The figure shows three views and two pictorial views of one solid part (mm, origin at its lowest corner). Answer the questions. A direction names the side the tool comes from. Give positions to 0.01 mm unless a question says otherwise; leave off trailing zeros. Write each loop counter-clockwise with the first axis right and the second up, starting at its lowest first coordinate (ties: lowest second). Pieces come first, ordered by that corner, then holes. Notation, with made-up numbers: (76, -16.5) -> (102, -16.5) arc R23 cw to (102, -0.5) -> close; hole circle Ø6 at (31, 26). An arc over 180 degrees is marked (long way). Answer as CSV lines item,"result". Start each with the question number.
1. The part is cut by section B-B, the plane x = 40. Determine the outline of the cut face in (y, z), and give its area (3 significant figures).
2. The part is cut by section A-A, the plane y = 40. Determine the outline of the cut face in (x, z).
3. The part is cut by section C-C, the plane z = 2. Determine the outline of the cut face in (x, y).
4. Given pin 1 (4 mm diameter, centred on x = 60.5, z = 7.5, fed in from +Y); pin 2 (8 mm diameter, centred on x = 49.5, y = 11, fed in from +Z); pin 3 (10 mm diameter, centred on x = 66, z = 3.5, fed in from -Y), each flat-ended and moving along its own axis, determine where each tip first touches the part or whether it passes through.
5. A tool of negligible diameter and unlimited length cuts with its end or side. For the marked faces 1 and 2, from which of +Z, -Z, +X, -X, +Y, -Y can it reach the whole face along a straight path? Write none if from no direction.
6. Find the intervals of material crossed by line 1 (Y direction, x = 40, z = 7.5); line 2 (Z direction, x = 40, y = 35); line 3 (Z direction, x = 74, y = 21), in increasing order.
7. The part is cut by section D-D, the plane x = 20. Determine the outline of the cut face in (y, z), and give its area (4 significant figures).
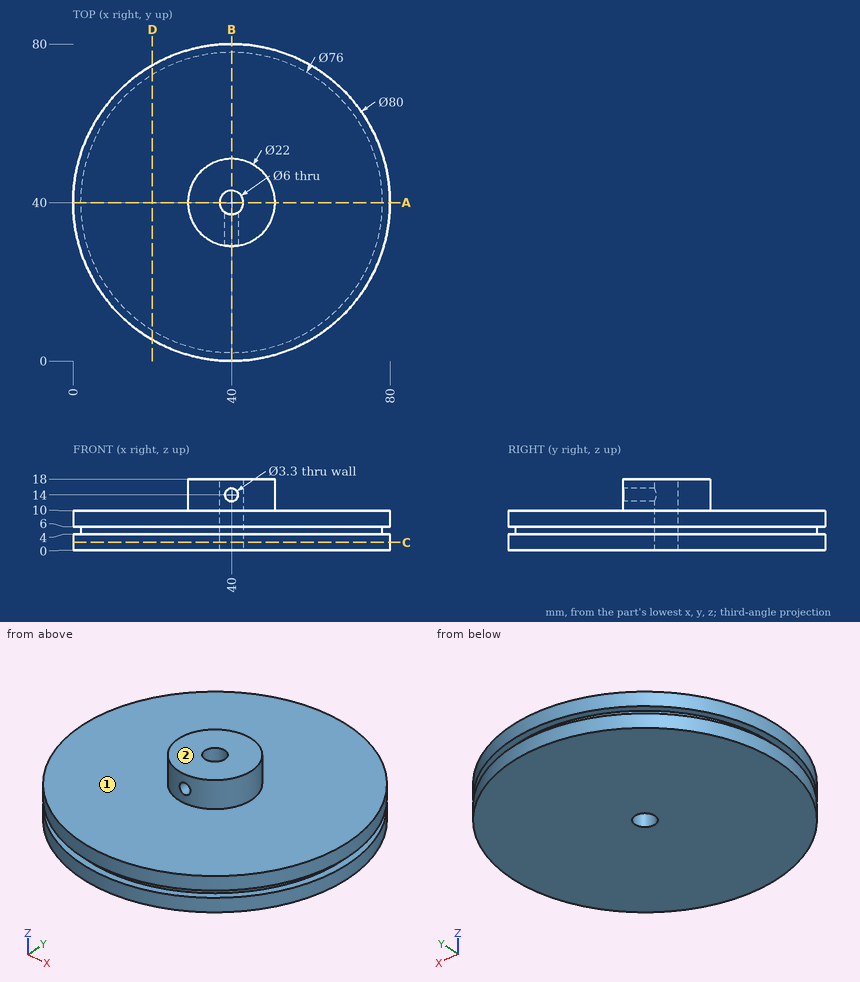
Results found:
1,outline,"(0, 0) -> (37, 0) -> (37, 12.35) -> (29, 12.35) -> (29, 10) -> (0, 10) -> (0, 6) -> (2, 6) -> (2, 4) -> (0, 4) -> close; (29, 15.65) -> (37, 15.65) -> (37, 18) -> (29, 18) -> close; (43, 0) -> (80, 0) -> (80, 4) -> (78, 4) -> (78, 6) -> (80, 6) -> (80, 10) -> (51, 10) -> (51, 18) -> (43, 18) -> close"
1,area,"834 mm²"
2,outline,"(0, 0) -> (37, 0) -> (37, 18) -> (29, 18) -> (29, 10) -> (0, 10) -> (0, 6) -> (2, 6) -> (2, 4) -> (0, 4) -> close; (43, 0) -> (80, 0) -> (80, 4) -> (78, 4) -> (78, 6) -> (80, 6) -> (80, 10) -> (51, 10) -> (51, 18) -> (43, 18) -> close"
3,outline,"circle Ø80 at (40, 40); hole circle Ø6 at (40, 40)"
4,pin 1,"stops at y = 75.46"
4,pin 2,"stops at z = 10"
4,pin 3,"stops at y = 5.96"
5,face 1,"+Z"
5,face 2,"+Z, +X, -X, +Y, -Y"
6,line 1,"y = 0 to 37, 43 to 80"
6,line 2,"z = 0 to 12.35, 15.65 to 18"
6,line 3,"z = 0 to 4, 6 to 10"
7,outline,"(5.36, 0) -> (74.64, 0) -> (74.64, 4) -> (72.31, 4) -> (72.31, 6) -> (74.64, 6) -> (74.64, 10) -> (5.36, 10) -> (5.36, 6) -> (7.69, 6) -> (7.69, 4) -> (5.36, 4) -> close"
7,area,"683.5 mm²"
